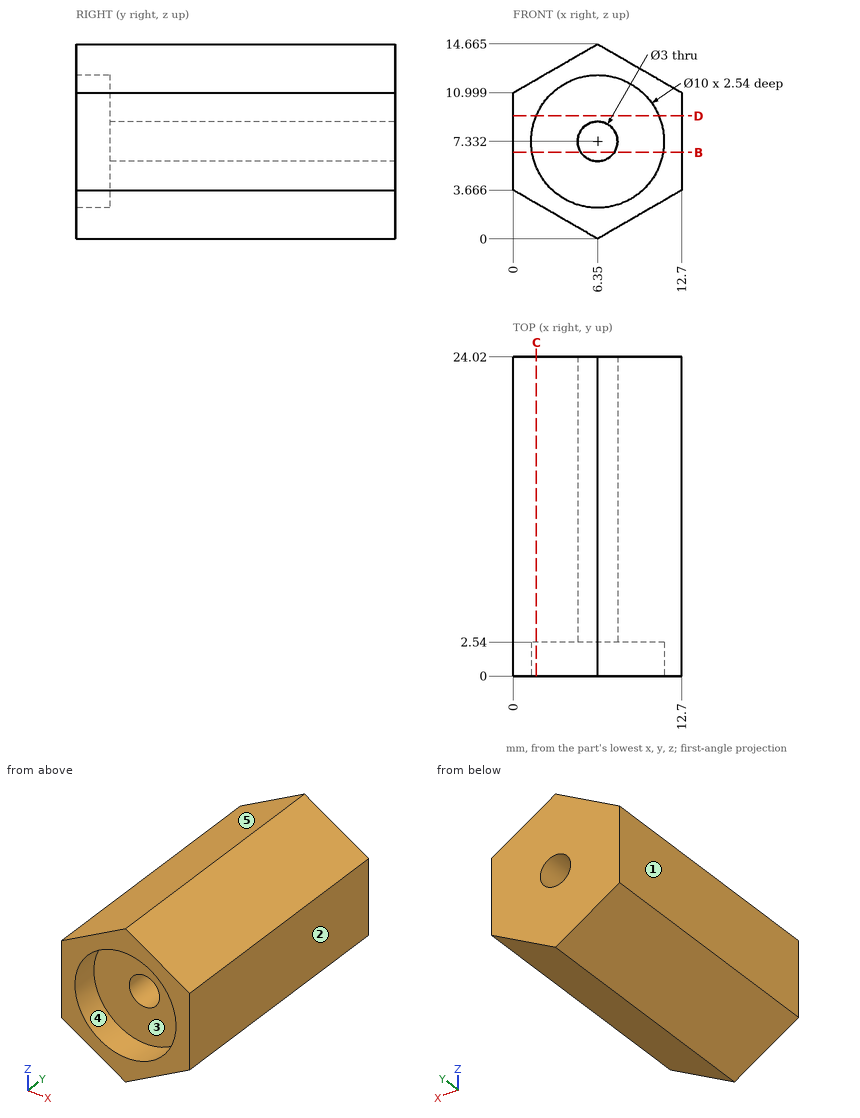
The drawing under review shows one solid part. Ordinate dimensions are in mm from its lowest x, y, z. A direction names the side the tool comes from. Round coordinates to 2 decimals unless told otherwise and drop trailing zeros. Write each loop counter-clockwise with the first axis right and the second up, starting at its lowest first coordinate (ties: lowest second). Pieces come first, ordered by that corner, then holes. Notation, with made-up numbers: (17.25, -7) - (67.25, -7) arc R20 cw to (67.25, 1) - close; hole circle Ø5 at (-13, 73). An arc over 180 degrees is marked (long way). Write each question's results on one line, items separated by ' | '.
Item 1: Draft analysis for pull direction X (two halves, no side actions). For the marked faces 1, 2 and 3, state which applies: pulls with the +X half, pulls with the -X half, needs draft (parallel to the pull), parting line crosses it, or undercut.
Calculated:
face 1: pulls with the -X half | face 2: pulls with the +X half | face 3: undercut
Item 2: Take a section at C-C on x = 1.75. State the section outline as (y, z) points (1 decimal).
Calculated:
outline: (0, 2.7) - (24, 2.7) - (24, 12) - (0, 12) - (0, 9.3) - (2.5, 9.3) - (2.5, 5.4) - (0, 5.4) - close
Item 3: To check wall thickness, follow line 1 along X through (y, z) = (10.25, 7.25); line 2 along Y through (x, z) = (7, 3.25); line 3 along X through (y, z) = (6.25, 8) (1 decimal). State the ranges of each line that lie inside material, in increasing order. Write a range as from..to.
Calculated:
line 1: x = 0..4.85, 7.85..12.7 | line 2: y = 2.54..24.02 | line 3: x = 0..5, 7.7..12.7
Item 4: For the marked faces 4 and 5, list the 3-axis set-ups (+Z, -Z, +X, -X, +Y, -Y) from which the entire face can be reached by the end or side of a thin tool; tool diameter is ignored.
Calculated:
face 4: -Y | face 5: +Z, -X, +Y, -Y
Item 5: For pin 1 (5 mm diameter, centred on x = 2.5, z = 13, fed in from +Y); pin 2 (1.5 mm diameter, centred on y = 19.5, z = 12, fed in from +X) (1 decimal); pin 3 (5 mm diameter, centred on x = 6, y = 7, fed in from -Z); pin 4 (2.5 mm diameter, centred on x = 6.35, z = 7.33, fed in from -Y), all flat-tipped, find the tip position at first contact; note any pin that passes through.
Calculated:
pin 1: stops at y = 24.02 | pin 2: stops at x = 12.3 | pin 3: stops at z = 0 | pin 4: passes through
Item 6: Take a section at D-D on z = 9.25. State the section outline as (x, y) points, then the cut area to 3 significant figures.
Calculated:
outline: (0, 0) - (1.73, 0) - (1.73, 2.54) - (10.97, 2.54) - (10.97, 0) - (12.7, 0) - (12.7, 24.02) - (0, 24.02) - close | area: 282 mm^2
Item 7: Take a section at B-B on z = 6.5. State the section outline as (x, y) points.
Calculated:
outline: (0, 0) - (1.42, 0) - (1.42, 2.54) - (5.1, 2.54) - (5.1, 24.02) - (0, 24.02) - close; (7.6, 2.54) - (11.28, 2.54) - (11.28, 0) - (12.7, 0) - (12.7, 24.02) - (7.6, 24.02) - close
